Part model, mm, in its own coordinate system. Face numbers are marked on the shaded views. A direction names the side the tool comes from. Give positions to 0.01 mm unless a question says otherwise; leave off trailing zeros. Order: outer loops, then holes, each group sorted by start corner. A loop starts at its lowest first (then second) coordinate and runs counter-clockwise, first axis right, second up. Notation, with made-up numbers: M 82,89 L 100,89 A35 cw 100,122 Z; hole C 70.25,82.5 d1. An arc over 180 degrees is marked long. Return JSON: item names as keys, results as strings.
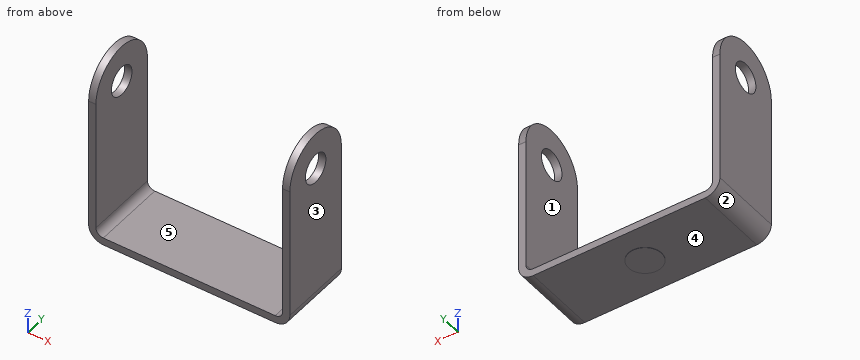
Autodesk Inventor part; units mm, degrees
ref_plane "YZ Plane" through (0, 0, 0) normal (1, 0, 0) x (0, 1, 0)
ref_plane "XZ Plane" through (0, 0, 0) normal (0, 1, 0) x (-1, 0, 0)
ref_plane "XY Plane" through (0, 0, 0) normal (0, 0, 1) x (1, 0, 0)
sketch "Sketch1" plane through (0, 0, 0) normal (0, 0, 1) x (1, 0, 0)
  line L0 (0, 0) -> (27.5, 0)
  line L1 (27.5, -20) -> (0, -20)
  line L2 (0, 0) -> (0, -20)
  line L3 (0, 0) -> (-27.5, 0)
  line L4 (-27.5, -20) -> (0, -20)
  line L5 (27.5, 0) -> (27.5, -20)
  line L6 (-27.5, 0) -> (-27.5, -20)
  dimension "d0" = 27.5
  dimension "d6" = 20
extrude "Extrusion1" add sketch "Sketch1" along normal mid plane 2
sketch "Sketch2" plane through (-25.5, -20, -1) normal (-1, 0, 0) x (0, -1, 0)
  line L0 (-20, 0) -> (0, 0)
  line L1 (0, 0) -> (0, 50)
  line L2 (0, 50) -> (-20, 50)
  line L3 (-20, 50) -> (-20, 0)
edge flange "Flange1" height 50 angle 90 thickness 2 bend radius 2 thickness toward (-1, 0, 0) relief tear relief width 2 relief depth 1 edges at (-27.5, -10, 1) wall of the first edge with corners at (-25.5, 0, -1) (-25.5, -20, -1) (-25.5, -20, 49) (-25.5, 0, 49)
bend "Bend1"
corner "Corner1"
sketch "Sketch3" plane through (25.5, 0, -1) normal (1, 0, 0) x (0, 1, 0)
  line L0 (-20, 0) -> (0, 0)
  line L1 (0, 0) -> (0, 50)
  line L2 (0, 50) -> (-20, 50)
  line L3 (-20, 50) -> (-20, 0)
edge flange "Flange2" height 50 angle 90 thickness 2 bend radius 2 thickness toward (1, 0, 0) relief tear relief width 2 relief depth 1 edges at (27.5, -10, 1) wall of the first edge with corners at (25.5, -20, -1) (25.5, 0, -1) (25.5, 0, 49) (25.5, -20, 49)
bend "Bend2"
corner "Corner2"
sketch "Sketch5" plane through (27.5, -20, 49) normal (1, 0, 0) x (0, 0, -1)
  line L0 (46, 0) -> (0, 0)
  line L1 (0, 0) -> (0, 20)
  line L2 (0, 20) -> (0, 0)
  line L3 (0, 0) -> (0, 20)
  line L4 (0, 20) -> (10, 20)
  line L5 (0, 0) -> (10, 0)
  line L6 (0, 0) -> (46, 0)
  arc A0 (10, 20) -> (10, 0) centre (10, 10) ccw
  line L7 (0, 20) -> (46, 20)
  circle A1 centre (10, 10) radius 4
  point P0 (49, 20)
  point P1 (0, 10)
  dimension "d38" = 10
  dimension "d39" = 10
  dimension "d40" = 10
  dimension "d46" = 8
extrude "Cut1" cut sketch "Sketch5" against normal blind 2
sketch "Sketch6" plane through (-27.5, -20, 49) normal (-1, 0, 0) x (0, 0, 1)
  line L0 (0, 20) -> (0, 0)
  line L1 (-10, 0) -> (0, 0)
  line L2 (0, 0) -> (0, 20)
  line L3 (0, 20) -> (-10, 20)
  line L4 (-46, 20) -> (0, 20)
  arc A0 (-10, 0) -> (-10, 20) centre (-10, 10) ccw
  circle A1 centre (-10, 10) radius 4
  point P0 (-49, 20)
  point P1 (0, 10)
  dimension "d43" = 10
  dimension "d47" = 8
extrude "Cut2" cut sketch "Sketch6" against normal blind 2
sketch "Sketch7" plane through (0, 0, -1) normal (0, 0, -1) x (-1, 0, 0)
  line L0 (23.5, 0) -> (-23.5, 0)
  line L1 (-23.5, -20) -> (23.5, -20)
  circle A0 centre (0, -10) radius 4.5
  line L2 (23.5, -20) -> (23.5, 0)
  line L3 (-23.5, 0) -> (-23.5, -20)
  point P0 (0, 0)
  dimension "d48" = 10
  dimension "d49" = 9
  dimension "d53" = 23.5
extrude "Extrusion2" add sketch "Sketch7" along normal blind 0.1 contours A0
equation "\"d41\" = Thickness"
equation "\"d44\" = Thickness"
equation "\"d7\" = Thickness"
equation "\"d8\" = BendReliefWidth"
equation "\"d9\" = BendReliefDepth"
equation "\"d10\" = MinimumRemnant"
equation "\"d11\" = TransitionRadius"
equation "\"d14\" = BendRadius"
equation "\"d15\" = CornerReliefSize"
equation "\"d16\" = GapSize"
equation "\"d17\" = JacobiRadiusSize"
equation "\"d18\" = BendReliefWidth"
equation "\"d19\" = BendReliefDepth"
equation "\"d20\" = MinimumRemnant"
equation "\"d21\" = TransitionRadius"
equation "\"d24\" = BendRadius"
equation "\"d25\" = CornerReliefSize"
equation "\"d26\" = GapSize"
equation "\"d27\" = JacobiRadiusSize"
equation "\"BendRadius\" = Thickness"
equation "\"BendReliefWidth\" = Thickness"
equation "\"BendReliefDepth\" = 0.5 * Thickness"
equation "\"CornerReliefSize\" = 4 * Thickness"
equation "\"MinimumRemnant\" = 2 * Thickness"
equation "\"TransitionRadius\" = BendRadius"
equation "\"JacobiRadiusSize\" = BendRadius"
equation "\"GapSize\" = Thickness"
properties part number "SHEET_METAL1"
Q1. Probe line 1 along X through (y, z) = (-11.5, 25); line 2 along Y through (x, z) = (26, 39); line 3 along Z through (x, y) = (4.5, -17.5). List the from-to ranges inside material, lowest first.
Established:
{"line 1": "x = -27.5 to -25.5, 25.5 to 27.5", "line 2": "y = -20 to -14, -6 to 0", "line 3": "z = -1 to 1"}
Q2. Band-saw the part on B-B (y = -10). Give the cut face in (x, z).
Established:
{"outline": "M -27.5,3 A4 ccw -23.5,-1 L -4.5,-1 L -4.5,-1.1 L 4.5,-1.1 L 4.5,-1 L 23.5,-1 A4 ccw 27.5,3 L 27.5,35 L 25.5,35 L 25.5,3 A2 cw 23.5,1 L -23.5,1 A2 cw -25.5,3 L -25.5,35 L -27.5,35 Z; M -27.5,43 L -25.5,43 L -25.5,49 L -27.5,49 Z; M 25.5,43 L 27.5,43 L 27.5,49 L 25.5,49 Z"}
Q3. Band-saw the part on D-D (y = -16.75). Give the cut face in (x, z).
Established:
{"outline": "M -27.5,3 A4 ccw -23.5,-1 L 23.5,-1 A4 ccw 27.5,3 L 27.5,46.38 L 25.5,46.38 L 25.5,3 A2 cw 23.5,1 L -23.5,1 A2 cw -25.5,3 L -25.5,46.38 L -27.5,46.38 Z"}
Q4. Pin check, flat tips, straight feed: pin 1 (10.5 mm diameter, centred on y = -10, z = 39, fed in from +X); pin 2 (6 mm diameter, centred on x = 7.5, y = -13.5, fed in from +Z); pin 3 (3 mm diameter, centred on x = -22, y = -13, fed in from -Z). Stop position of each tip, or through.
Established:
{"pin 1": "stops at x = 27.5", "pin 2": "stops at z = 1", "pin 3": "stops at z = -1"}
Q5. 3-axis set-ups, long thin cutter, end or side, ignore diameter. For the marked faces 1 and 2: which of +Z, -Z, +X, -X, +Y, -Y reach the whole face in a straight line?
Established:
{"face 1": "+Z, +Y, -Y", "face 2": "-Z, -X, +Y, -Y"}
Q6. Band-saw the part on A-A (z = 17). Give the cut face in (x, y), then the cut area to 3 significant figures.
Established:
{"outline": "M -27.5,-20 L -25.5,-20 L -25.5,0 L -27.5,0 Z; M 25.5,-20 L 27.5,-20 L 27.5,0 L 25.5,0 Z", "area": "80.0 mm²"}
Q7. Two-plate mould, pull along X, no slides. Class the marked faces 3, 4 and 5: +X half, -X half, draft (parallel to the pull), parting line (faces both ways), or undercut.
Established:
{"face 3": "+X half", "face 4": "draft", "face 5": "undercut"}
Q8. Band-saw the part on C-C (x = 0). Give the cut face in (y, z).
Established:
{"outline": "M -20,-1 L -14.5,-1 L -14.5,-1.1 L -5.5,-1.1 L -5.5,-1 L 0,-1 L 0,1 L -20,1 Z"}
